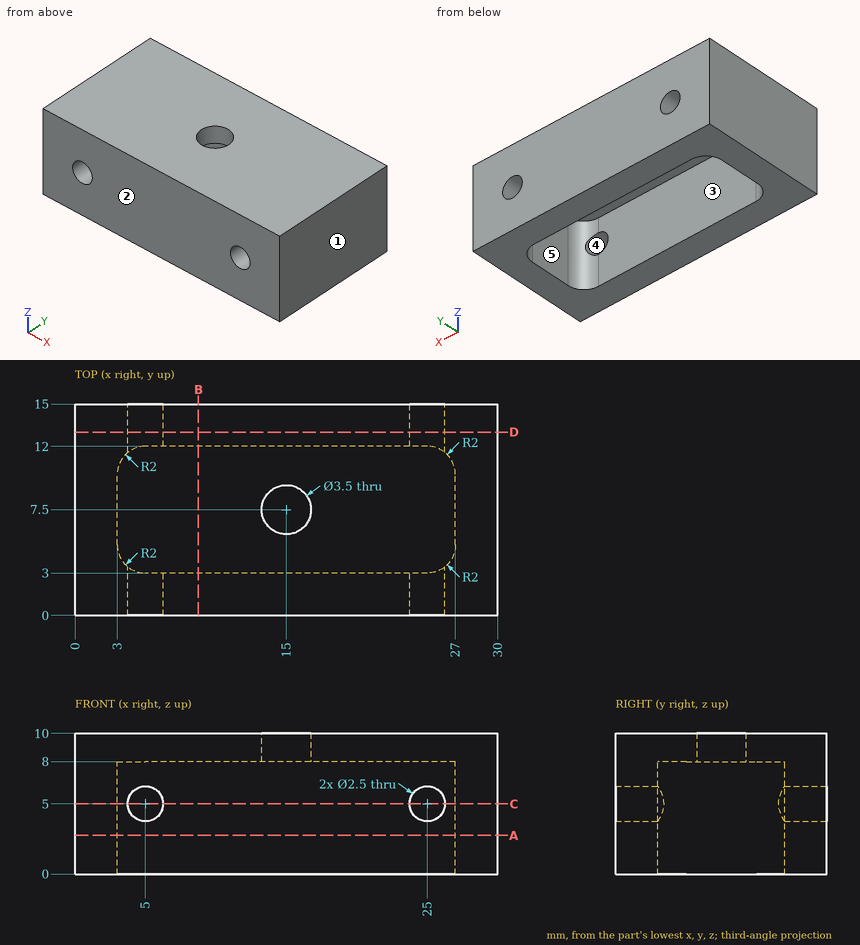
Geometry: see drawing. Coordinates: mm, zero at the bounding-box minimum. A direction names the side the tool comes from. Round coordinates to 2 decimals unless told otherwise and drop trailing zeros. Loops run counter-clockwise (first coordinate to the right, second up) from the corner with the lowest first, then second, coordinate; pieces in that order, holes last. Notation, with made-up numbers: (81.25, 8) -> (89.25, 8) arc R33 cw to (89.25, 36) -> close; hole circle Ø10 at (21.5, 7). An arc over 180 degrees is marked (long way). Write each question's results on one line, items separated by ' | '.
Item 1: Pull-direction query (Y, two-part tool) for the marked faces 1, 2 and 3; classes: pulls with the +Y half, pulls with the -Y half, needs draft (parallel to the pull), parting line crosses it, or undercut.
Answers below:
face 1: needs draft | face 2: pulls with the -Y half | face 3: undercut
Item 2: Cut plane B-B on x = 8.75. Return the cut outline in (y, z), and give its area (3 significant figures).
Answers below:
outline: (0, 0) -> (3, 0) -> (3, 8) -> (12, 8) -> (12, 0) -> (15, 0) -> (15, 10) -> (0, 10) -> close | area: 78.0 mm²
Item 3: Cut plane A-A on z = 2.75. Return the cut outline in (x, y), and give its area (3 significant figures).
Answers below:
outline: (0, 0) -> (30, 0) -> (30, 15) -> (0, 15) -> close; hole (3, 5) arc R2 ccw to (5, 3) -> (25, 3) arc R2 ccw to (27, 5) -> (27, 10) arc R2 ccw to (25, 12) -> (5, 12) arc R2 ccw to (3, 10) -> close | area: 237 mm²
Item 4: Set-up query: the marked faces 4 and 5. Return all of +Z, -Z, +X, -X, +Y, -Y with unobstructed straight access to the full face (end or side cutting, diameter ignored); none if empty.
Answers below:
face 4: +Y, -Y | face 5: -Z
Item 5: Cut plane D-D on y = 13. Return the cut outline in (x, z).
Answers below:
outline: (0, 0) -> (30, 0) -> (30, 10) -> (0, 10) -> close; hole circle Ø2.5 at (5, 5); hole circle Ø2.5 at (25, 5)
Item 6: Pin query (flat end, axial travel): pin 1 Ø4 at (x, y) = (25.5, 8) entering from -Z; pin 2 Ø2.5 at (x, y) = (20.5, 6.5) entering from -Z. Return the tip coordinate at first contact, or that it passes through.
Answers below:
pin 1: stops at z = 0 | pin 2: stops at z = 8
Item 7: Line query: probe 1 along Y at (x, z) = (11.5, 5.5); probe 2 along X at (y, z) = (9, 6); probe 3 along Y at (x, z) = (15, 8.9). Output: solid intervals per line, ascending. Write a range as [from, to].
Answers below:
probe 1: y = [0, 3], [12, 15] | probe 2: x = [0, 3], [27, 30] | probe 3: y = [0, 5.75], [9.25, 15]
Item 8: Cut plane C-C on z = 5. Return the cut outline in (x, y), and give its area (3 significant figures).
Answers below:
outline: (0, 0) -> (3.75, 0) -> (3.75, 3.44) arc R2 cw to (3, 5) -> (3, 10) arc R2 cw to (3.75, 11.56) -> (3.75, 15) -> (0, 15) -> close; (6.25, 0) -> (23.75, 0) -> (23.75, 3) -> (6.25, 3) -> close; (6.25, 12) -> (23.75, 12) -> (23.75, 15) -> (6.25, 15) -> close; (26.25, 0) -> (30, 0) -> (30, 15) -> (26.25, 15) -> (26.25, 11.56) arc R2 cw to (27, 10) -> (27, 5) arc R2 cw to (26.25, 3.44) -> close | area: 207 mm²
